Could you check a few things on this model? Use its own coordinates, in mm. A direction names the side the tool comes from. Coordinates: 2 decimals unless noted, no trailing zeros. Loops run counter-clockwise (first coordinate to the right, second up) from the corner with the lowest first, then second, coordinate; pieces in that order, holes last. Notation, with made-up numbers: (-24, 12.5) - (16, 12.5) arc R29 ccw to (16, 48.5) - close; hole circle Ø1 at (72, 86). An arc over 180 degrees is marked (long way). One line per item, written item: value. Start each with the question number.
(1) If we section it at A-A on x = -11.5: Write out the boundary of the cut face in (y, z), then the cut area to 3 significant figures.
(2) If we section it at C-C on x = 18.5: Write out the boundary of the cut face in (y, z).
(3) I'm going to push flat-ended pins straight in: P1, Ø10, axis at y = -1, z = 57, coming from the +X side; P2, Ø9, axis at x = 12.5, z = 69, coming from the -Y side; P3, Ø2.5, axis at y = -7, z = 20.5, coming from the -X side; P4, Ø10, axis at y = -33, z = 64.5, coming from the -X side. Where does each tip first touch, or does it pass through?
(4) If we section it at D-D on z = 40: Write out the boundary of the cut face in (x, y).
(5) If we mould it in two halves opening along X, with no side actions, what happens to faces 1 (the face through (4, 35, 65)), 2 (the face through (-12, 20, 47.5)), 3 (the face through (22.983, -43.494, 20.035))? For each: pulls with the +X half, pulls with the -X half, needs draft (parallel to the pull), parting line crosses it, or undercut.
(6) On a 3-axis mill with a long thin cutter (end or side, diameter ignored), from which of +Z, -Z, +X, -X, +Y, -Y can I reach the whole of each face in a straight line? I mean faces 4 (the face through (44.347, 4.034, 70.07)), 5 (the face through (0, 20, 37)), 6 (the face through (23, 0, 9)), 7 (the face through (-12, 20, 17.5)). Say none if no direction works.
(7) If I drill on line 1 along Y through (x, z) = (4.5, 69.75); line 2 along Y through (x, z) = (23.5, 69.5); line 3 along Z through (x, y) = (14.5, -28), over which ranges is the centre line in solid material (lowest first)? Write a range as from..to.
(8) If we section it at B-B on z = 54.5: Write out the boundary of the cut face in (x, y), then the cut area to 3 significant figures.
```python
from build123d import *

# Parameters (mm, degrees)
SZKIC1_W                    = 47
SZKIC1_H                    = 39.6
DODANIE_WYCI_GNI_CIE3_DEPTH = 75
SZKIC4_R                    = 8.15
DODANIE_WYCI_GNI_CIE4_DEPTH = 10
SZKIC5_R                    = 8.15
DODANIE_WYCI_GNI_CIE5_DEPTH = 5
SZKIC6_R                    = 2
WYTNIJ_WYCI_GNI_CIE1_DEPTH  = 10


with BuildPart() as part:
    # Szkic1 → Dodanie-wyciągnięcie3 (new body)
    with BuildSketch(Plane.XY):
        with Locations((23.5, 19.8)):
            Rectangle(SZKIC1_W, SZKIC1_H)
    extrude(amount=DODANIE_WYCI_GNI_CIE3_DEPTH)

    # Szkic4 → Dodanie-wyciągnięcie4 (add)
    with BuildSketch(Plane(origin=(0, 0, 27.5), x_dir=(-1, 0, 0), z_dir=(0, 0, -1))):
        with BuildLine():
            Line((-47, 39.6), (-72.479949748, 39.6))
            ThreePointArc((-72.479949748, 39.6), (-88.399748742, 18), (-68.5, 0))
            Line((-68.5, 0), (-47, 0))
            Line((-47, 0), (-47, 39.6))
        make_face()
        with Locations((-68.5, 20)):
            Circle(SZKIC4_R, mode=Mode.SUBTRACT)
        with BuildLine():
            Line((21.5, 0), (0, 0))
            Line((0, 0), (0, 39.6))
            Line((0, 39.6), (25.479949748, 39.6))
            ThreePointArc((25.479949748, 39.6), (41.399748742, 18), (21.5, 0))
        make_face()
        with Locations((21.5, 20)):
            Circle(SZKIC4_R, mode=Mode.SUBTRACT)
    dodanie_wyci_gni_cie4 = extrude(amount=DODANIE_WYCI_GNI_CIE4_DEPTH)

    # Lustro1: Dodanie-wyciągnięcie4 across plane
    add(dodanie_wyci_gni_cie4.mirror(Plane(origin=(0, 0, 37.5), x_dir=(1, 0, 0), z_dir=(0, 0, -1))))

    # Szkic5 → Dodanie-wyciągnięcie5 (add)
    with BuildSketch(Plane(origin=(0, 0, 22.5), x_dir=(-1, 0, 0), z_dir=(0, 0, -1))):
        with BuildLine():
            Line((-47, 0), (0, 0))
            Line((0, 0), (0, -20))
            ThreePointArc((0, -20), (-23.5, -43.5), (-47, -20))
            Line((-47, -20), (-47, 0))
        make_face()
        with Locations((-23.5, -20)):
            Circle(SZKIC5_R, mode=Mode.SUBTRACT)
    dodanie_wyci_gni_cie5 = extrude(amount=DODANIE_WYCI_GNI_CIE5_DEPTH)

    # Lustro2: Dodanie-wyciągnięcie5 across plane
    add(dodanie_wyci_gni_cie5.mirror(Plane(origin=(0, 0, 37.5), x_dir=(1, 0, 0), z_dir=(0, 0, -1))))

    # Szkic6 → Wytnij-wyciągnięcie1 (cut)
    with BuildSketch(Plane.XY.offset(75)):
        with Locations((4.5, 4.8)):
            Circle(SZKIC6_R)
        with Locations((4.5, 34.8)):
            Circle(SZKIC6_R)
        with Locations((42.5, 34.8)):
            Circle(SZKIC6_R)
        with Locations((42.5, 4.8)):
            Circle(SZKIC6_R)
        with Locations((23.5, 32.8)):
            Circle(SZKIC6_R)
        with Locations((23.5, 6.8)):
            Circle(SZKIC6_R)
    extrude(amount=-WYTNIJ_WYCI_GNI_CIE1_DEPTH, mode=Mode.SUBTRACT)


solid = part.part
```
Values:
1. outline: (0, 17.5) - (39.6, 17.5) - (39.6, 27.5) - (0, 27.5) - close; (0, 47.5) - (39.6, 47.5) - (39.6, 57.5) - (0, 57.5) - close
1. area: 792 mm2
2. outline: (-42.96, 17.5) - (-26.44, 17.5) - (-26.44, 22.5) - (-42.96, 22.5) - close; (-42.96, 52.5) - (-26.44, 52.5) - (-26.44, 57.5) - (-42.96, 57.5) - close; (-13.56, 17.5) - (0, 17.5) - (0, 0) - (39.6, 0) - (39.6, 75) - (0, 75) - (0, 57.5) - (-13.56, 57.5) - (-13.56, 52.5) - (0, 52.5) - (0, 22.5) - (-13.56, 22.5) - close
3. P1: stops at x = 80.5
3. P2: stops at y = 0
3. P3: stops at x = 0
3. P4: passes through
4. outline: (0, 0) - (47, 0) - (47, 39.6) - (0, 39.6) - close
5. face 1: undercut
5. face 2: needs draft
5. face 3: parting line crosses it
6. face 4: +Z
6. face 5: -X, +Y, -Y
6. face 6: -Z, +X, -X, -Y
6. face 7: -Z, -X, +Y, -Y
7. line 1: y = 0..2.8, 6.8..32.8, 36.8..39.6
7. line 2: y = 0..4.8, 8.8..30.8, 34.8..39.6
7. line 3: z = 17.5..22.5, 52.5..57.5
8. outline: (-25.48, 39.6) arc R20 ccw to (-21.5, 0) - (0, 0) - (0, -20) arc R23.5 ccw to (47, -20) - (47, 0) - (68.5, 0) arc R20 ccw to (72.48, 39.6) - close; hole circle Ø16.3 at (-21.5, 20); hole circle Ø16.3 at (23.5, -20); hole circle Ø16.3 at (68.5, 20)
8. area: 6,000 mm2
